Read the model definition and answer for the solid it produces. Units are mm, in the model's axes. A direction names the side the tool comes from. Give positions to 0.01 mm unless a question says otherwise; leave off trailing zeros. Write each loop counter-clockwise with the first axis right and the second up, starting at its lowest first coordinate (ties: lowest second). Pieces come first, ordered by that corner, then holes.
Autodesk Inventor part; units mm, degrees
ref_plane "YZ Plane" through (0, 0, 0) normal (1, 0, 0) x (0, 1, 0)
ref_plane "XZ Plane" through (0, 0, 0) normal (0, 1, 0) x (-1, 0, 0)
ref_plane "XY Plane" through (0, 0, 0) normal (0, 0, 1) x (1, 0, 0)
sketch "Szkic1" plane through (0, 0, 0) normal (0, 0, 1) x (1, 0, 0)
  line L0 (-15, -2) -> (15, -2)
  line L1 (15, -2) -> (15, 2)
  line L2 (15, 2) -> (5, 2)
  line L3 (-15, 2) -> (-15, -2)
  line L4 (-15, -2) -> (15, 2) construction
  line L5 (15, -2) -> (-15, 2) construction
  line L6 (-5, 2) -> (-0.75, 2)
  line L7 (5, 2) -> (5, 19.755)
  line L8 (5, 22) -> (-5, 22)
  line L9 (-5, 22) -> (-5, 2)
  line L10 (-0.75, 28.2995) -> (0.75, 28.2995)
  line L11 (0.75, 28.2995) -> (0.75, 33.9648)
  line L12 (0.75, 35.6626) -> (-0.75, 35.6626)
  line L13 (-0.75, 35.6626) -> (-0.75, 33.9648)
  line L14 (-0.75, 28.2995) -> (0.75, 35.6626) construction
  line L15 (0.75, 28.2995) -> (-0.75, 35.6626) construction
  line L16 (-0.75, 33.9648) -> (-0.75, 28.2995)
  arc A0 (5, 19.755) -> (0.75, 33.9648) centre (0, 26) ccw
  arc A1 (0.9, 22) -> (0.75, 30.0308) centre (0, 26) ccw
  arc A2 (-0.75, 30.0308) -> (0.9, 22) centre (0, 26) ccw
  arc A3 (-0.75, 33.9648) -> (-5, 19.755) centre (0, 26) ccw
  line L17 (0.75, 33.9648) -> (0.75, 35.6626)
  arc A4 (-5, 19.755) -> (2.749, 18.4871) centre (0, 26) ccw
  arc A5 (2.749, 18.4871) -> (5, 19.755) centre (0, 26) ccw
  line L18 (5, 19.755) -> (5, 22)
  line L19 (5, 2) -> (-15, 2)
  line L20 (-0.75, 2) -> (5, 2)
  point P0 (0, 0)
  point P1 (0, 31.981)
  dimension "d0" = 30
  dimension "d1" = 4
  dimension "d2" = 10
  dimension "d3" = 20
  dimension "d4" = 5
  dimension "d6" = 4
  dimension "d7" = 5
  dimension "d9" = 1.5
  dimension "d10" = 7.3631
  dimension "d11" = 31.981
  dimension "d12" = 5
  dimension "d13" = 8
  dimension "d14" = 4.1
extrude "Wyciągnięcie proste1" add sketch "Szkic1" against normal blind 8 contours L3 L19 L6 L2 L1 L0 | L9 A4 A5 L7 L19 L6 | A3 L16 A2 L8 L9 | L9 L8 A2 L18 A5 A4 | L18 L8 A1 L11 A0
sketch "Szkic2" plane through (0, 0, -8) normal (0, 0, -1) x (-1, 0, 0)
  line L0 (-15, 2) -> (15, 2)
  line L1 (15, 2) -> (15, -2)
  line L2 (15, -2) -> (-15, -2)
  line L3 (-15, -2) -> (-15, 2)
  point P0 (0, 0)
extrude "Wyciągnięcie proste2" add sketch "Szkic2" along normal blind 7
sketch "Szkic3" plane through (-0.75, 30.0308, 0) normal (1, 0, 0) x (0, 0, -1)
  line L0 (0, 3.9339) -> (0, 0)
  line L1 (0, 0) -> (8, 0)
  line L2 (8, 0) -> (8, 9)
  line L3 (8, 9) -> (0, 9)
  line L4 (0, 9) -> (0, 0)
  point P0 (0, -30.0308)
  dimension "d19" = 8
  dimension "d20" = 9
extrude "Wyciągnięcie proste3" add sketch "Szkic3" against normal blind 3
sketch "Szkic4" plane through (-3.75, 30.0308, 0) normal (-1, 0, 0) x (0, 0, 1)
  line L0 (0, 9) -> (-8, 9)
  line L1 (0, 3.0358) -> (0, 9)
  point P0 (0, -30.0308)
  point P1 (-4, 6)
  dimension "d23" = 3
  dimension "d24" = 4
hole "Otwór1" at (-3.75, 36.0308, -4) direction (1, 0, 0) diameter 3 depth 8 tip angle 118
mirror "Odbij1" about plane through (0, 0, 0) normal (1, 0, 0) of "Wyciągnięcie proste3", "Otwór1"
sketch "Szkic5" plane through (0, 0, -8) normal (0, 0, -1) x (-1, 0, 0)
  arc A0 (-3.75, 33.0666) -> (-5, 19.755) centre (0, 26) ccw
  line L0 (5, 2) -> (15, 2)
  line L1 (-5, 19.755) -> (5, 19.755)
  line L2 (5, 19.755) -> (5, 2)
  line L3 (5, 2) -> (-5, 2)
  line L4 (-5, 2) -> (-5, 19.755)
  point P0 (0, 0)
extrude "Wyciągnięcie proste4" add sketch "Szkic5" along normal blind 7
sketch "Szkic7" plane through (-5, 2, 0) normal (-1, 0, 0) x (0, 0, 1)
  line L0 (0, 17.755) -> (-8, 17.755)
  line L1 (-15, -4) -> (-15, 0)
  line L2 (-8, 17.755) -> (-15, 0)
  line L3 (-15, 17.755) -> (-15, 0)
  line L4 (-15, 0) -> (-15, 17.755)
  line L5 (-8, 17.755) -> (-15, 17.755)
  line L6 (-15, 17.755) -> (-8, 17.755)
  point P0 (0, -2)
extrude "Wyciągnięcie proste5" cut sketch "Szkic7" against normal through all
sketch "Szkic8" plane through (-15, 2, 0) normal (0, 1, 0) x (1, 0, 0)
  line L0 (0, 0) -> (0, 15)
  line L1 (0, 15) -> (10, 15)
  line L2 (15, 0) -> (15, 15) construction
  point P0 (5, 7.5)
  point P1 (25, 7.5)
  dimension "d36" = 5
  dimension "d37" = 7.5
hole "Otwór2" at (-10, 2, -7.5) at (10, 2, -7.5) direction (0, -1, 0) diameter 3 depth 8 tip angle 118
properties part number "Kamera_uchwyt" material "Tworzywo sztuczne PET"
Item 1: Section C-C (y = 28.5) is taken. Write down the section's boundary in (x, z), and give its area (3 significant figures).
Result set:
outline: (-7.6, -8) - (-3.25, -8) - (-3.25, 0) - (-7.6, 0) - close; (3.25, -8) - (7.6, -8) - (7.6, 0) - (3.25, 0) - close
area: 69.6 mm2
Item 2: Section D-D (z = -7.5) is taken. Write down the section's boundary in (x, y) (3 decimals), and give its area (3 significant figures).
Result set:
outline: (-15, -2) - (-11.5, -2) - (-11.5, 2) - (-15, 2) - close; (-8.5, -2) - (8.5, -2) - (8.5, 2) - (5, 2) - (5, 19.755) arc R8 ccw to (3.75, 33.067) - (3.75, 39.031) - (0.75, 39.031) - (0.75, 30.031) arc R4.1 cw to (0.9, 22) arc R4.1 cw (long way) to (-0.75, 30.031) - (-0.75, 39.031) - (-3.75, 39.031) - (-3.75, 33.067) arc R8 ccw to (-5, 19.755) - (-5, 2) - (-8.5, 2) - close; (11.5, -2) - (15, -2) - (15, 2) - (11.5, 2) - close
area: 436 mm2
Item 3: Which of the six approach directions +Z, -Z, +X, -X, +Y, -Y give full straight-line access (tool end or side, diameter ignored) to faces 1 (the flat face through (5, 11, -6)), 2 (the flat face through (-3.75, 37.42, -3.06)), 3 (the flat face through (-9.9, 2, -5.7)), 4 (the flat face through (3.75, 37.42, -4.94))?
Result set:
face 1: +Z, -Z, +X
face 2: +Z, -Z, -X, +Y
face 3: +Z, -Z, -X
face 4: +Z, -Z, +X, +Y
Item 4: Section A-A (z = -4) is taken. Write down the section's boundary in (x, y) (3 decimals).
Result set:
outline: (-15, -2) - (15, -2) - (15, 2) - (5, 2) - (5, 19.755) arc R8 ccw to (3.75, 33.067) - (3.75, 34.531) - (0.75, 34.531) - (0.75, 30.031) arc R4.1 cw to (0.9, 22) arc R4.1 cw (long way) to (-0.75, 30.031) - (-0.75, 34.531) - (-3.75, 34.531) - (-3.75, 33.067) arc R8 ccw to (-5, 19.755) - (-5, 2) - (-15, 2) - close; (-3.75, 37.531) - (-0.75, 37.531) - (-0.75, 39.031) - (-3.75, 39.031) - close; (0.75, 37.531) - (3.75, 37.531) - (3.75, 39.031) - (0.75, 39.031) - close
Item 5: Section B-B (x = 10) is taken. Write down the section's boundary in (y, z), and give its area (3 significant figures).
Result set:
outline: (-2, -15) - (2, -15) - (2, -9) - (-2, -9) - close; (-2, -6) - (2, -6) - (2, 0) - (-2, 0) - close
area: 48.0 mm2
Item 6: Find the intervals of material crossed by line 1 along Z through (x, y) = (10, -1); line 2 along Y through (x, z) = (2.4, -4); line 3 along Y through (x, z) = (12.5, -1.75), in increasing order.
Result set:
line 1: z = -15 to -9, -6 to 0
line 2: y = -2 to 22.68, 29.32 to 34.53, 37.53 to 39.03
line 3: y = -2 to 2
Item 7: Each of these flat-tipped pins is pushed along its axis until it touches: pin 1 Ø8 at (x, y) = (-1, 25) entering from -Z; pin 2 Ø2.5 at (y, z) = (36.03, -4) entering from -X; pin 3 Ø2 at (x, z) = (11.5, -1.5) entering from +Y; pin 4 Ø3 at (y, z) = (37.5, -5) entering from -X. Where does it stop, or does it pass through?
Result set:
pin 1: stops at z = -8
pin 2: passes through
pin 3: stops at y = 2
pin 4: stops at x = -3.75
Item 8: Determine the mould class of faces 5 (the cylindrical face through (7.975, 26.638, -3.944)), 6 (the flat face through (0, -2, -7)), 7 (the flat face through (0.75, 34, -4)) for opening direction X: pulls with the +X half, pulls with the -X half, needs draft (parallel to the pull), parting line crosses it, or undercut.
Result set:
face 5: pulls with the +X half
face 6: needs draft
face 7: undercut
